Source: CAD feature listing. Evaluate the final solid. Frame: model axes, mm. Face numbers are marked on the shaded views. A direction names the side the tool comes from. Give positions to 0.01 mm unless a question says otherwise; leave off trailing zeros. Write each loop counter-clockwise with the first axis right and the second up, starting at its lowest first coordinate (ties: lowest second). Pieces come first, ordered by that corner, then holes. Notation, with made-up numbers: (20.25, -35) -> (76.25, -35) arc R22 ccw to (76.25, 3) -> close; hole circle Ø2 at (11, 3). An arc over 180 degrees is marked (long way). Use a Markdown table: item, result. Add a question column.
```python
from build123d import *

# Parameters (mm, degrees)
SKETCH1_W           = 100
SKETCH1_H           = 50
SKETCH1_R           = 1.5
SKETCH1_R_2         = 2
SKETCH1_R_3         = 2.5
SKETCH1_R_4         = 3
SKETCH1_R_5         = 3.5
SKETCH1_R_6         = 4
SKETCH1_R_7         = 4.5
SKETCH1_R_8         = 5
BOSS_EXTRUDE1_DEPTH = 20
CUT_EXTRUDE2_DEPTH  = 114.578166916


with BuildPart() as part:
    # Sketch1 → Boss-Extrude1 (new body)
    with BuildSketch(Plane(origin=(0, 0, 0), x_dir=(1, 0, 0), z_dir=(0, 1, 0))):
        with Locations((50, 25)):
            Rectangle(SKETCH1_W, SKETCH1_H)
        with Locations(Location((10, 25, 0), (0, 0, 270))):
            Circle(SKETCH1_R, mode=Mode.SUBTRACT)
        with Locations(Location((20, 25, 0), (0, 0, 270))):
            Circle(SKETCH1_R_2, mode=Mode.SUBTRACT)
        with Locations(Location((30, 25, 0), (0, 0, 270))):
            Circle(SKETCH1_R_3, mode=Mode.SUBTRACT)
        with Locations(Location((40, 25, 0), (0, 0, 270))):
            Circle(SKETCH1_R_4, mode=Mode.SUBTRACT)
        with Locations(Location((50, 25, 0), (0, 0, 270))):
            Circle(SKETCH1_R_5, mode=Mode.SUBTRACT)
        with Locations(Location((60, 25, 0), (0, 0, 270))):
            Circle(SKETCH1_R_6, mode=Mode.SUBTRACT)
        with Locations(Location((72, 25, 0), (0, 0, 270))):
            Circle(SKETCH1_R_7, mode=Mode.SUBTRACT)
        with Locations(Location((87, 25, 0), (0, 0, 270))):
            Circle(SKETCH1_R_8, mode=Mode.SUBTRACT)
    extrude(amount=BOSS_EXTRUDE1_DEPTH)

    # Sketch2 → Cut-Extrude2 (cut, through all)
    with BuildSketch(Plane(origin=(100, 0, 0), x_dir=(0, 0, -1), z_dir=(1, 0, 0))):
        Polygon((15, 0), (25, 10), (35, 0), align=None)
    extrude(amount=-CUT_EXTRUDE2_DEPTH, mode=Mode.SUBTRACT)


solid = part.part
```
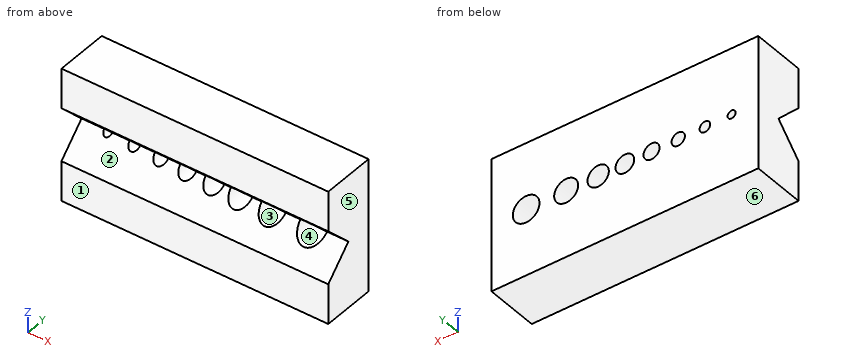
(1) Cut plane B-B on y = 13. Count the separate pieces of the cut face and the enclosed holes in it, then the cut area to 3 significant figures.
(2) Cut plane A-A on x = 20. Return the cut outline in (y, z).
(3) First-contact query: pin 1 Ø9 at (x, z) = (60, -25) entering from -Y; pin 2 Ø7 at (x, z) = (40, -25) entering from -Y; pin 3 Ø1 at (x, z) = (57.5, -33) entering from -Y. Flat tips, straight axial feed; report the tip coordinate or a pass-through.
(4) Access query for the marked faces 1 and 2. Directions: +Z, -Z, +X, -X, +Y, -Y. A direction counts if a zero-diameter tool reaches every point of the face in a straight line with its end or side. Return the directions, or none.
(5) Mould query, pull axis Z, two halves, no side actions, for the marked faces 3, 4, 5 and 6. Classes: +Z half, -Z half, draft (parallel to the pull), parting line (faces both ways), or undercut.
(6) Cut plane D-D on x = 60. Return the cut outline in (y, z), then the cut area to 3 significant figures.
(7) Material intervals for L1, parallel to Z at x = 20, y = 11.75; L2, parallel to Z at x = 72, y = 12.5; L3, parallel to Y at x = 79.5, z = -27, sorted ascending.
(8) Cut plane C-C on x = 93. Return the cut outline in (y, z), then the cut area to 3 significant figures.
Output:
| question | item | result |
|---|---|---|
| 1 | separate pieces | 1 |
| 1 | enclosed holes | 8 |
| 1 | area | 4,700 mm^2 |
| 2 | outline | (0, -50) -> (20, -50) -> (20, -27) -> (8, -27) -> (0, -35) -> close; (0, -15) -> (8, -23) -> (20, -23) -> (20, 0) -> (0, 0) -> close |
| 3 | pin 1 | y = 5.5 |
| 3 | pin 2 | y = 6.5 |
| 3 | pin 3 | y = 1.5 |
| 4 | face 1 | +Z, -Z, +X, -X, -Y |
| 4 | face 2 | +X, -X, -Y |
| 5 | face 3 | undercut |
| 5 | face 4 | undercut |
| 5 | face 5 | draft |
| 5 | face 6 | -Z half |
| 6 | outline | (0, -50) -> (20, -50) -> (20, -29) -> (6, -29) -> (0, -35) -> close; (0, -15) -> (6, -21) -> (20, -21) -> (20, 0) -> (0, 0) -> close |
| 6 | area | 804 mm^2 |
| 7 | L1 | -50 to -27, -23 to 0 |
| 7 | L2 | -50 to -29.5, -20.5 to 0 |
| 7 | L3 | 8 to 20 |
| 8 | outline | (0, -50) -> (20, -50) -> (20, 0) -> (0, 0) -> (0, -15) -> (10, -25) -> (0, -35) -> close |
| 8 | area | 900 mm^2 |
